Verification items for the finished model (mm, model axes). Face numbers are marked on the shaded views. A direction names the side the tool comes from. Give positions to 0.01 mm unless a question says otherwise; leave off trailing zeros. Write each loop counter-clockwise with the first axis right and the second up, starting at its lowest first coordinate (ties: lowest second). Pieces come first, ordered by that corner, then holes. Notation, with made-up numbers: M 33,77.5 L 83,77.5 A34 ccw 83,116.5 Z; hole C 44,-33 d10. An arc over 180 degrees is marked long. Answer as a JSON object with one key per item and string values.
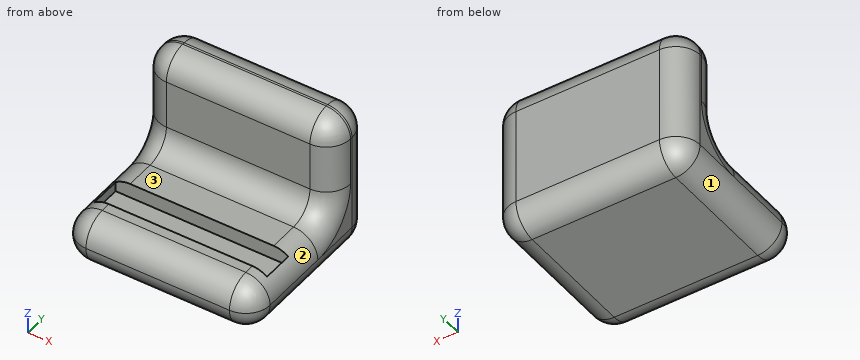
```python
from build123d import *

# Parameters (mm, degrees)
F0_W         = 100.5891636014
F0_H         = 89.0790522099
F1_DEPTH     = 25.4
F2_W         = 100.5891636014
F2_H         = 26.5494063497
F3_DEPTH     = 50.8
F4_W         = 90.4291636014
F4_H         = 16.5267549455
F5_DEPTH     = 7.62
F6_F1_R      = 12.7
F6_F2_R      = 12.6999
F6_T3_DEPTH  = 49.8296458602
F6_T5_DEPTH  = 38.1
F6_T8_ANGLE  = 90
F6_T10_ANGLE = 90
F6_T12_ANGLE = 90
F6_T14_ANGLE = 90
F6_T16_ANGLE = 90
F6_T18_ANGLE = 90


# Not quite as in the source:
# - a fillet or chamfer that OpenCascade refuses, or shapes differently, is made with other operations: its cross-section is extruded or revolved along the edge and cut away or added
# - a fillet or chamfer is up to 0.001 mm smaller than in the source, because OpenCascade refuses the exact size


with BuildPart() as f1:
    # F0 (on Top) → F1 (new body)
    with BuildSketch(Plane.XY):
        with Locations((1.1365450919, 10.1573467255)):
            Rectangle(F0_W, F0_H)
    extrude(amount=F1_DEPTH)

    # F2 (on face) → F3 (join)
    with BuildSketch(Plane.XY.offset(25.4)):
        with Locations((1.1365450919, 41.4221696556)):
            Rectangle(F2_W, F2_H)
    extrude(amount=F3_DEPTH)

    # F4 (on face) → F5 (cut)
    with BuildSketch(Plane.XY.offset(25.4)):
        with Locations((1.1365450919, -8.2633774728)):
            Rectangle(F4_W, F4_H)
    extrude(amount=-F5_DEPTH, mode=Mode.SUBTRACT)

    # F6: fillet of radius 12.7 on 18 edges, made by hand

    # F6_f1
    f6_f1_edges = [f1.edges().sort_by_distance(p)[0] for p in [
        (1.1365450919, 28.1474664807, 25.4),
    ]]
    fillet(f6_f1_edges, radius=F6_F1_R)

    # F6_f2 (radius 12.7 in the source; OpenCascade refuses exactly that, so slightly less here)
    f6_f2_edges = [f1.edges().sort_by_distance(p)[0] for p in [
        (1.1365450919, -34.3821793795, 25.4),
        (51.4311268926, -34.3821793795, 12.7),
        (1.1365450919, -34.3821793795, 0),
        (-49.1580367088, -34.3821793795, 12.7),
        (1.1365450919, 28.1474664807, 76.2),
        (51.4311268926, 10.1573467255, 0),
        (51.4311268926, 54.6968728304, 38.1),
        (51.4311268926, 41.4221696556, 76.2),
        (1.1365450919, 54.6968728304, 76.2),
        (-49.1580367088, 41.4221696556, 76.2),
        (-49.1580367088, 10.1573467255, 0),
        (-49.1580367088, 54.6968728304, 38.1),
        (1.1365450919, 54.6968728304, 0),
    ]]
    fillet(f6_f2_edges, radius=F6_F2_R)

    # F6_s4 → F6_t3 (cut)
    with BuildSketch(Plane.XZ.offset(-15.4474664807)):
        with BuildLine():
            ThreePointArc((-49.1580367088, 12.7), (-45.4382928299, 21.6802561211), (-36.4580367088, 25.4))
            Line((-36.4580367088, 25.4), (-36.4580367088, 25.654))
            Line((-36.4580367088, 25.654), (-49.4120367088, 25.654))
            Line((-49.4120367088, 25.654), (-49.4120367088, 12.7))
            Line((-49.4120367088, 12.7), (-49.1580367088, 12.7))
        make_face()
        with BuildLine():
            ThreePointArc((38.7311268926, 25.4), (47.7113830136, 21.6802561211), (51.4311268926, 12.7))
            Line((51.4311268926, 12.7), (51.6851268926, 12.7))
            Line((51.6851268926, 12.7), (51.6851268926, 25.654))
            Line((51.6851268926, 25.654), (38.7311268926, 25.654))
            Line((38.7311268926, 25.654), (38.7311268926, 25.4))
        make_face()
    extrude(amount=F6_T3_DEPTH, mode=Mode.SUBTRACT)

    # F6_s6 → F6_t5 (cut)
    with BuildSketch(Plane.XY.offset(38.1)):
        with BuildLine():
            ThreePointArc((-49.1580367088, 40.8474664807), (-45.4382928299, 31.8672103597), (-36.4580367088, 28.1474664807))
            Line((-36.4580367088, 28.1474664807), (-36.4580367088, 27.8934664807))
            Line((-36.4580367088, 27.8934664807), (-49.4120367088, 27.8934664807))
            Line((-49.4120367088, 27.8934664807), (-49.4120367088, 40.8474664807))
            Line((-49.4120367088, 40.8474664807), (-49.1580367088, 40.8474664807))
        make_face()
        with BuildLine():
            ThreePointArc((38.7311268926, 28.1474664807), (47.7113830136, 31.8672103597), (51.4311268926, 40.8474664807))
            Line((51.4311268926, 40.8474664807), (51.6851268926, 40.8474664807))
            Line((51.6851268926, 40.8474664807), (51.6851268926, 27.8934664807))
            Line((51.6851268926, 27.8934664807), (38.7311268926, 27.8934664807))
            Line((38.7311268926, 27.8934664807), (38.7311268926, 28.1474664807))
        make_face()
    extrude(amount=F6_T5_DEPTH, mode=Mode.SUBTRACT)

    # F6_s7 → F6_t8 (revolve, cut)
    with BuildSketch(Plane.XY.offset(12.7)):
        with BuildLine():
            ThreePointArc((38.7312268926, -34.3821793795), (47.711412303, -30.6624647899), (51.4311268926, -21.6822793795))
            Line((51.4311268926, -21.6822793795), (51.4311268926, -34.3821793795))
            Line((51.4311268926, -34.3821793795), (38.7312268926, -34.3821793795))
        make_face()
    revolve(axis=Axis((38.7311268926, -34.3821793795, 12.7), (0, -1, 0)), revolution_arc=F6_T8_ANGLE, mode=Mode.SUBTRACT)

    # F6_s9 → F6_t10 (revolve, cut)
    with BuildSketch(Plane.YZ.offset(38.7311268926)):
        with BuildLine():
            ThreePointArc((40.8473664807, 76.2), (31.8671810703, 72.4802854104), (28.1474664807, 63.5001))
            Line((28.1474664807, 63.5001), (28.1474664807, 76.2))
            Line((28.1474664807, 76.2), (40.8473664807, 76.2))
        make_face()
    revolve(axis=Axis((38.7311268926, 40.8474664807, 76.2), (0, 0, 1)), revolution_arc=F6_T10_ANGLE, mode=Mode.SUBTRACT)

    # F6_s11 → F6_t12 (revolve, cut)
    with BuildSketch(Plane.XZ.offset(-40.8474664807)):
        with BuildLine():
            ThreePointArc((-36.4581367088, 76.2), (-45.4383221192, 72.4802854104), (-49.1580367088, 63.5001))
            Line((-49.1580367088, 63.5001), (-49.1580367088, 76.2))
            Line((-49.1580367088, 76.2), (-36.4581367088, 76.2))
        make_face()
    revolve(axis=Axis((-36.4580367088, 40.8474664807, 76.2), (0, 0, 1)), revolution_arc=F6_T12_ANGLE, mode=Mode.SUBTRACT)

    # F6_s13 → F6_t14 (revolve, cut)
    with BuildSketch(Plane.YZ.offset(-36.4580367088)):
        with BuildLine():
            ThreePointArc((-34.3821793795, 12.7001), (-30.6624647899, 21.6802854104), (-21.6822793795, 25.4))
            Line((-21.6822793795, 25.4), (-34.3821793795, 25.4))
            Line((-34.3821793795, 25.4), (-34.3821793795, 12.7001))
        make_face()
    revolve(axis=Axis((-36.4580367088, -34.3821793795, 12.7), (0, -1, 0)), revolution_arc=F6_T14_ANGLE, mode=Mode.SUBTRACT)

    # F6_s15 → F6_t16 (revolve, cut)
    with BuildSketch(Plane.XY.offset(38.1)):
        with BuildLine():
            ThreePointArc((38.7311268926, 28.1474664807), (47.7113830136, 31.8672103597), (51.4311268926, 40.8474664807))
            Line((51.4311268926, 40.8474664807), (51.6851268926, 40.8474664807))
            Line((51.6851268926, 40.8474664807), (51.6851268926, 27.8934664807))
            Line((51.6851268926, 27.8934664807), (38.7311268926, 27.8934664807))
            Line((38.7311268926, 27.8934664807), (38.7311268926, 28.1474664807))
        make_face()
    revolve(axis=Axis((51.4311268926, 15.4474664807, 38.1), (-1, 0, 0)), revolution_arc=F6_T16_ANGLE, mode=Mode.SUBTRACT)

    # F6_s17 → F6_t18 (revolve, cut)
    with BuildSketch(Plane.XY.offset(38.1)):
        with BuildLine():
            ThreePointArc((-49.1580367088, 40.8474664807), (-45.4382928299, 31.8672103597), (-36.4580367088, 28.1474664807))
            Line((-36.4580367088, 28.1474664807), (-36.4580367088, 27.8934664807))
            Line((-36.4580367088, 27.8934664807), (-49.4120367088, 27.8934664807))
            Line((-49.4120367088, 27.8934664807), (-49.4120367088, 40.8474664807))
            Line((-49.4120367088, 40.8474664807), (-49.1580367088, 40.8474664807))
        make_face()
    revolve(axis=Axis((-49.1580367088, 15.4474664807, 38.1), (-1, 0, 0)), revolution_arc=F6_T18_ANGLE, mode=Mode.SUBTRACT)


solid = f1.part
```
1) Thickness scan on L1, parallel to Y at x = -24, z = 39; L2, parallel to Z at x = -14.5, y = -17.5; L3, parallel to Z at x = 22, y = -11.5. Record the ranges inside material, lowest first.
Completed:
{"L1": "y = 28.15 to 54.7", "L2": "z = 0 to 25.4", "L3": "z = 0 to 17.78"}
2) Go/stop test with flat-tipped pins: pin 1 (18 mm diameter, centred on x = -4.5, y = -8, fed in from +Z); pin 2 (1.5 mm diameter, centred on y = -15, z = 8, fed in from +X); pin 3 (5.5 mm diameter, centred on y = -4, z = 20.5, fed in from -X). Record where each tip stops, or that it passes through.
Completed:
{"pin 1": "stops at z = 25.4", "pin 2": "stops at x = 50.8", "pin 3": "stops at x = -48.11"}
3) Section check A-A on z = 57. Record the boundary of the cut face in (x, y), and give its area (3 significant figures).
Completed:
{"outline": "M -49.16,40.85 A12.7 ccw -36.46,28.15 L 38.73,28.15 A12.7 ccw 51.43,40.85 L 51.43,42 A12.7 ccw 38.73,54.7 L -36.46,54.7 A12.7 ccw -49.16,42 Z", "area": "2,530 mm2"}
4) Access from +Z, -Z, +X, -X, +Y, -Y to the whole of each face (thin tool, end or side, straight path). Record for the marked faces 1, 2 and 3.
Completed:
{"face 1": "-Z, -X, +Y, -Y", "face 2": "+Z, +X, -Y", "face 3": "+Z, +X, -X, -Y"}
